from build123d import *

# Parameters (mm, degrees)
BOSS_EXTRUDE1_DEPTH      = 40
BOSS_EXTRUDE1_DEPTH_BACK = 40
CUT_EXTRUDE1_DEPTH       = 68.268120235
CUT_EXTRUDE1_DEPTH_BACK  = 68.268120235


with BuildPart() as part:
    # Sketch3 → Boss-Extrude1 (new, two sides: drawn at the far end of the back side and taken through both)
    with BuildSketch(Plane(origin=(0, 0, 0), x_dir=(0, 0, -1), z_dir=(1, 0, 0)).offset(-BOSS_EXTRUDE1_DEPTH_BACK)):
        Polygon((-30, -15.5), (-23, -22.5), (30, -22.5), (30, 22.5), (-23, 22.5), (-30, 15.5), align=None)
    extrude(amount=BOSS_EXTRUDE1_DEPTH + BOSS_EXTRUDE1_DEPTH_BACK)

    # Sketch4 → Cut-Extrude1 (cut, two sides: drawn at the far end of the back side and taken through both)
    with BuildSketch(Plane(origin=(0, 22.5, 0), x_dir=(1, 0, 0), z_dir=(0, 1, 0)).offset(-CUT_EXTRUDE1_DEPTH_BACK)):
        with BuildLine():
            Line((18, 15), (-18, 15))
            ThreePointArc((-18, 15), (-22.949747468, 12.949747468), (-25, 8))
            Line((-25, 8), (-25, -30))
            Line((-25, -30), (25, -30))
            Line((25, -30), (25, 8))
            ThreePointArc((25, 8), (22.949747468, 12.949747468), (18, 15))
        make_face()
    extrude(amount=CUT_EXTRUDE1_DEPTH + CUT_EXTRUDE1_DEPTH_BACK, mode=Mode.SUBTRACT)


solid = part.part
Design review of the part built by this model. Coordinates are the model's own, in mm. A direction names the side the tool comes from. Round coordinates to 2 decimals unless told otherwise and drop trailing zeros. Loops run counter-clockwise (first coordinate to the right, second up) from the corner with the lowest first, then second, coordinate; pieces in that order, holes last. Notation, with made-up numbers: (32, -10.75) - (66, -10.75) arc R15 cw to (66, 18.25) - close; hole circle Ø11 at (20, 69.5). An arc over 180 degrees is marked (long way). One line per item, written item: value. Start each with the question number.
1) Consider section A-A on z = -5.5. Give the boundary of the cut face in (x, y), then the cut area to 3 significant figures.
2) Draft analysis for pull direction X (two halves, no side actions). For faces 1 (the flat face through (32.4, -19, 26.5)), 2 (the flat face through (40, 0, 0)), 3 (the flat face through (25, 0, 11)), state which applies: +X half, -X half, draft (parallel to the pull), parting line (faces both ways), or undercut.
3) Consider section B-B on y = -10. Give the boundary of the cut face in (x, z), then the cut area to 3 significant figures.
4) Consider section C-C on x = 12.5. Give the boundary of the cut face in (y, z), then the cut area to 3 significant figures.
5) Consider section D-D on y = 18. Give the boundary of the cut face in (x, z).
6) For faces 4 (the flat face through (-32.6, 19, 26.5)), 5 (the cylindrical face through (23, -0.3, -12.9)), list the 3-axis set-ups (+Z, -Z, +X, -X, +Y, -Y) from which the entire face can be reached by the end or side of a thin tool; tool diameter is ignored.
7) To check wall thickness, follow L1, parallel to X at y = -6, z = 23.5; L2, parallel to Z at x = 2, y = -18.5; L3, parallel to X at y = 9, z = -11.5. State the ranges of each line that lie inside material, in increasing order. Write a range as from..to.
8) Insertion check: pin 1 Ø12 at (x, y) = (-22, 3.5) entering from +Z. The pin has a flat end and moves straight along its axis. Give the tip position at first contact, or say it passes through.
Reported:
1. outline: (-40, -22.5) - (-25, -22.5) - (-25, 22.5) - (-40, 22.5) - close; (25, -22.5) - (40, -22.5) - (40, 22.5) - (25, 22.5) - close
1. area: 1,350 mm^2
2. face 1: draft
2. face 2: +X half
2. face 3: undercut
3. outline: (-40, -30) - (40, -30) - (40, 30) - (25, 30) - (25, -8) arc R7 cw to (18, -15) - (-18, -15) arc R7 cw to (-25, -8) - (-25, 30) - (-40, 30) - close
3. area: 2,570 mm^2
4. outline: (-22.5, -30) - (22.5, -30) - (22.5, -15) - (-22.5, -15) - close
4. area: 675 mm^2
5. outline: (-40, -30) - (40, -30) - (40, 27.5) - (25, 27.5) - (25, -8) arc R7 cw to (18, -15) - (-18, -15) arc R7 cw to (-25, -8) - (-25, 27.5) - (-40, 27.5) - close
6. face 4: +Z, +X, -X, +Y
6. face 5: +Z, +Y, -Y
7. L1: x = -40..-25, 25..40
7. L2: z = -30..-15
7. L3: x = -40..-24.06, 24.06..40
8. pin 1: stops at z = 30
